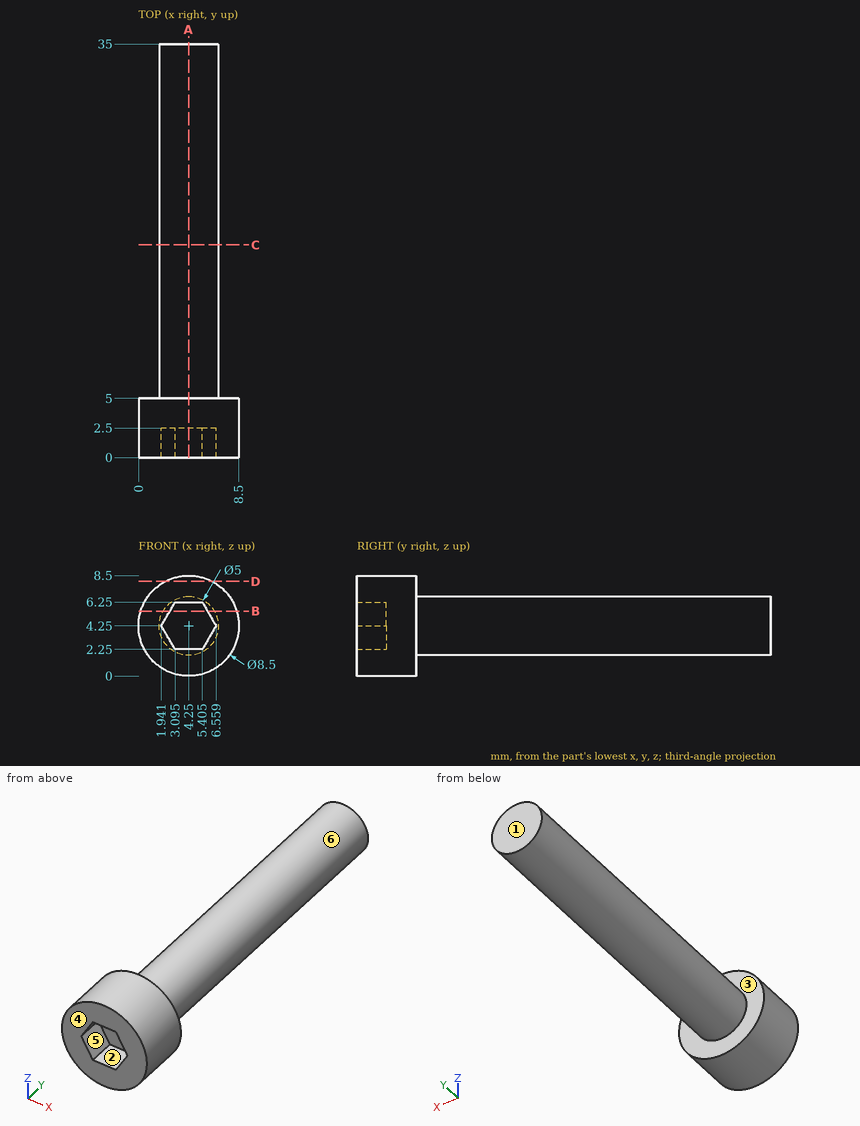
The drawing under review shows one solid part. Ordinate dimensions are in mm from its lowest x, y, z. A direction names the side the tool comes from. Give positions to 0.01 mm unless a question says otherwise; leave off trailing zeros. Order: outer loops, then holes, each group sorted by start corner. A loop starts at its lowest first (then second) coordinate and runs counter-clockwise, first axis right, second up. Notation, with made-up numbers: M 63,-0.5 L 78,-0.5 A20 ccw 78,6.5 Z; hole C 1,18 d11. An arc over 180 degrees is marked long. Answer in a Markdown table with one row per item. Add a question column.
1. To check wall thickness, follow line 1 along Z through (x, y) = (2.75, 10); line 2 along Y through (x, z) = (1.75, 2.25); line 3 along Z through (x, y) = (4.5, 3.5). State the ranges of each line that lie inside material, in increasing order.
2. Machinability: for the marked faces 1, 2 and 3, which of the approach directions +Z, -Z, +X, -X, +Y, -Y give a long, thin tool a straight path to every point of the face, cutting with its end or side? Answer none if there is none.
3. Add section D-D on z = 8. State the section outline as (x, y) points, plus the area to 3 significant figures.
4. Add section C-C on y = 18. State the section outline as (x, z) points, plus the area to 3 significant figures.
5. For pin 1 Ø4 at (x, y) = (1, 27) entering from +Z (1 decimal), flat-tipped, find the tip position at first contact; note if it passes through.
6. Add section B-B on z = 5.5. State the section outline as (x, y) points (1 decimal).
7. Add section A-A on x = 4.25. State the section outline as (y, z) points.
8. Mouldability with a two-part tool opening along Z and no side actions: class the marked faces 4, 5 and 6 as released by +Z, released by -Z, zero draft, split by the parting line, or undercut.
The answers:
| question | item | result |
|---|---|---|
| 1 | line 1 | 2.25 to 6.25 |
| 1 | line 2 | 0 to 5 |
| 1 | line 3 | 0.01 to 8.49 |
| 2 | face 1 | +Z, -Z, +X, -X, +Y |
| 2 | face 2 | -Y |
| 2 | face 3 | +Y |
| 3 | outline | M 2.25,0 L 6.25,0 L 6.25,5 L 2.25,5 Z |
| 3 | area | 20.0 mm2 |
| 4 | outline | C 4.25,4.25 d5 |
| 4 | area | 19.6 mm2 |
| 5 | pin 1 | z = 6.4 |
| 6 | outline | M 0.2,0 L 2.7,0 L 2.7,2.5 L 5.8,2.5 L 5.8,0 L 8.3,0 L 8.3,5 L 6.4,5 L 6.4,35 L 2.1,35 L 2.1,5 L 0.2,5 Z |
| 7 | outline | M 0,0 L 5,0 L 5,1.75 L 35,1.75 L 35,6.75 L 5,6.75 L 5,8.5 L 0,8.5 L 0,6.25 L 2.5,6.25 L 2.5,2.25 L 0,2.25 Z |
| 8 | face 4 | zero draft |
| 8 | face 5 | undercut |
| 8 | face 6 | split by the parting line |
